Work out the finished part from the listing and answer in its coordinate system (mm). A direction names the side the tool comes from. Round coordinates to 2 decimals unless told otherwise and drop trailing zeros. Write each loop counter-clockwise with the first axis right and the second up, starting at its lowest first coordinate (ties: lowest second). Pieces come first, ordered by that corner, then holes. Notation, with made-up numbers: (58, -13) -> (74, -13) arc R25 ccw to (74, 10) -> close; hole circle Ø6 at (2.5, 42.5). An arc over 180 degrees is marked (long way). Answer as a JSON object with one key per item and string values. Group by question number.
from build123d import *

# Parameters (mm, degrees)
SKETCH_R     = 1.5
PAD_DEPTH    = 5
SKETCH001_W  = 5
SKETCH001_H  = 11.4
PAD001_DEPTH = 25
SKETCH002_R  = 1.5
POCKET_DEPTH = 25.701


with BuildPart() as part:
    # Sketch → Pad (new body)
    with BuildSketch(Plane.XY):
        Polygon((0, 0), (0, 20), (30, 20), (30, 0), (20.7, 0), (20.7, 11.4), (9.3, 11.4), (9.3, 0), align=None)
        with Locations((4, 15)):
            Circle(SKETCH_R, mode=Mode.SUBTRACT)
        with Locations((26, 15)):
            Circle(SKETCH_R, mode=Mode.SUBTRACT)
    extrude(amount=PAD_DEPTH)

    # Sketch001 → Pad001 (new body)
    with BuildSketch(Plane.XY.offset(5)):
        with Locations((6.8, 5.7)):
            Rectangle(SKETCH001_W, SKETCH001_H)
        with Locations((23.2, 5.7)):
            Rectangle(SKETCH001_W, SKETCH001_H)
    extrude(amount=PAD001_DEPTH)

    # Sketch002 → Pocket (cut, through all)
    with BuildSketch(Plane.YZ.offset(25.7)):
        with Locations((5.7, 19)):
            Circle(SKETCH002_R)
        with Locations((5.7, 11)):
            Circle(SKETCH002_R)
    extrude(amount=-POCKET_DEPTH, mode=Mode.SUBTRACT)


solid = part.part
1) Straight lines are drawn through the part: L1, parallel to Z at x = 22.85, y = 5.7; L2, parallel to X at y = 3.25, z = 19.75; L3, parallel to Z at x = 1.75, y = 16. For each, find the intervals that lie inside material, in ascending order.
2) For a pull along Y with two mould halves and no side action, classify faces 6 (the face through (23.24, 7.13, 11.45)), 7 (the face through (7, 6, 30)), 8 (the face through (15, 20, 2)) as released by +Y, released by -Y, zero draft, split by the parting line, or undercut.
3) A cutting plane is placed at A-A on y = 2. Determine the outline of the cut face in (x, z), plus the area to 3 significant figures.
4) A cutting plane is placed at D-D on x = 7. Determine the outline of the cut face in (y, z).
5) A cutting plane is placed at B-B on z = 8.75. Determine the outline of the cut face in (x, y), plus the area to 3 significant figures.
6) Each of these flat-tipped pins is pushed along its axis until it touches: P1, Ø2.5, axis at x = 17, z = 3, coming from the -Y side; P2, Ø2.5, axis at x = 26, y = 15, coming from the +Z side; P3, Ø5, axis at x = 18.5, y = 18, coming from the +Z side; P4, Ø10, axis at x = 23, z = 6.5, coming from the -Y side. Where does it stop, or does it pass through?
7) A tool of negligible diameter and unlimited length cuts with its end or side. For faces 1 (the face through (7, 11.4, 17)), 2 (the face through (20.7, 6, 15)), 3 (the face through (25.7, 6, 17)), 4 (the face through (6.84, 7.13, 11.45)), 5 (the face through (4.3, 6, 17)), from which of +Z, -Z, +X, -X, +Y, -Y can it reach the whole face along a straight path? Write none if from no direction.
8) A cutting plane is placed at C-C on y = 5.7. Determine the outline of the cut face in (x, z).
Established:
{
 "1": {"L1": "z = 0 to 9.5, 12.5 to 17.5, 20.5 to 30", "L2": "x = 4.3 to 9.3, 20.7 to 25.7", "L3": "z = 0 to 5"},
 "2": {"face 6": "undercut", "face 7": "zero draft", "face 8": "released by +Y"},
 "3": {"outline": "(0, 0) -> (9.3, 0) -> (9.3, 30) -> (4.3, 30) -> (4.3, 5) -> (0, 5) -> close; (20.7, 0) -> (30, 0) -> (30, 5) -> (25.7, 5) -> (25.7, 30) -> (20.7, 30) -> close", "area": "343 mm²"},
 "4": {"outline": "(0, 0) -> (20, 0) -> (20, 5) -> (11.4, 5) -> (11.4, 30) -> (0, 30) -> close; hole circle Ø3 at (5.7, 11); hole circle Ø3 at (5.7, 19)"},
 "5": {"outline": "(4.3, 0) -> (9.3, 0) -> (9.3, 11.4) -> (4.3, 11.4) -> close; (20.7, 0) -> (25.7, 0) -> (25.7, 11.4) -> (20.7, 11.4) -> close", "area": "114 mm²"},
 "6": {"P1": "stops at y = 11.4", "P2": "passes through", "P3": "stops at z = 5", "P4": "stops at y = 0"},
 "7": {"face 1": "+Z, +X, -X, +Y", "face 2": "+Z, -Z, -Y", "face 3": "+Z, +X, +Y, -Y", "face 4": "+X, -X", "face 5": "+Z, -X, +Y, -Y"},
 "8": {"outline": "(0, 0) -> (9.3, 0) -> (9.3, 9.5) -> (4.3, 9.5) -> (4.3, 5) -> (0, 5) -> close; (4.3, 12.5) -> (9.3, 12.5) -> (9.3, 17.5) -> (4.3, 17.5) -> close; (4.3, 20.5) -> (9.3, 20.5) -> (9.3, 30) -> (4.3, 30) -> close; (20.7, 0) -> (30, 0) -> (30, 5) -> (25.7, 5) -> (25.7, 9.5) -> (20.7, 9.5) -> close; (20.7, 12.5) -> (25.7, 12.5) -> (25.7, 17.5) -> (20.7, 17.5) -> close; (20.7, 20.5) -> (25.7, 20.5) -> (25.7, 30) -> (20.7, 30) -> close"}
}
